Check sheet for the drawn part. Datum: minimum x, y, z corner. Units: mm. Round coordinates to 2 decimals unless told otherwise and drop trailing zeros. Write each loop counter-clockwise with the first axis right and the second up, starting at its lowest first coordinate (ties: lowest second). Pieces come first, ordered by that corner, then holes. Notation, with made-up numbers: (6, 72.25) - (53, 72.25) arc R10 ccw to (53, 76.25) - close; hole circle Ø10 at (86, 79). An arc over 180 degrees is marked (long way). Return JSON: item names as keys, results as strings. Group by question number.
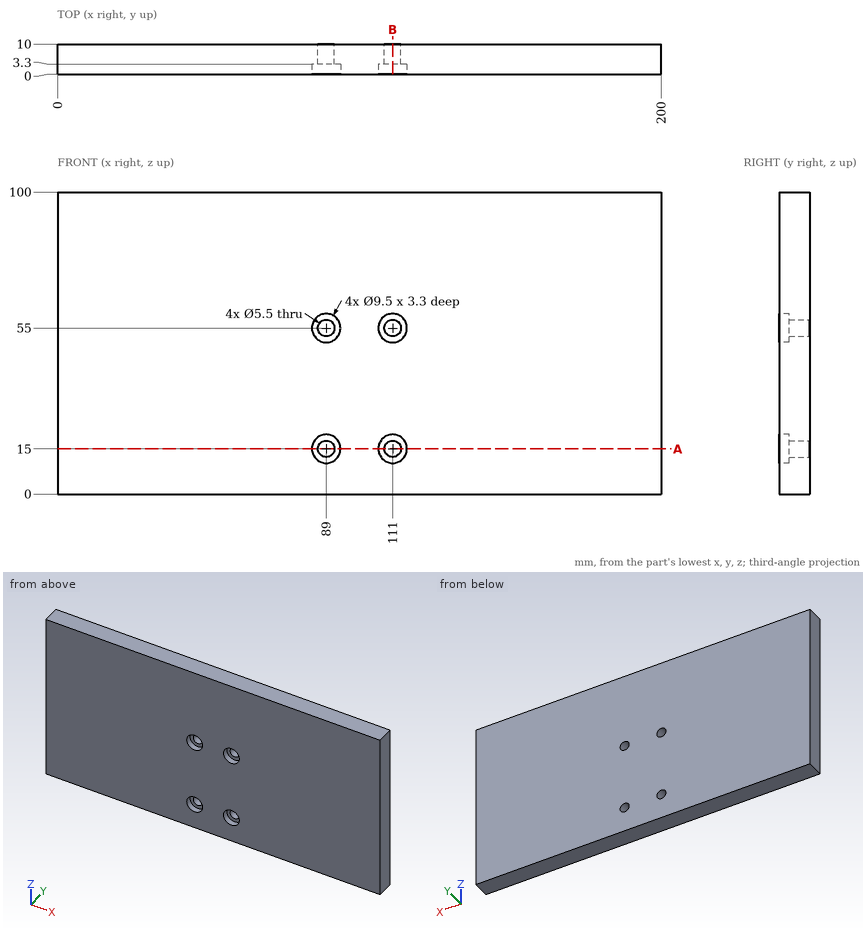
1. Section check A-A (z = 15). Enter the section's corners in (x, y).
2. Depth check by flat-ended pin: pin 1 Ø3.5 at (x, z) = (89, 55) entering from +Y; pin 2 Ø5 at (x, z) = (112, 14) entering from -Y. Enter the tip coordinate at first touch or a pass-through.
3. Material ranges on line 1 along X through (y, z) = (1, 15); line 2 along X through (y, z) = (3.5, 54); line 3 along Y through (x, z) = (113.5, 51), recorded low to high.
4. Section check B-B (x = 111). Enter the section's corners in (y, z), and give its area (3 significant figures).
Result sheet:
{
 "1": {"outline": "(0, 0) - (84.25, 0) - (84.25, 3.3) - (86.25, 3.3) - (86.25, 10) - (0, 10) - close; (91.75, 3.3) - (93.75, 3.3) - (93.75, 0) - (106.25, 0) - (106.25, 3.3) - (108.25, 3.3) - (108.25, 10) - (91.75, 10) - close; (113.75, 3.3) - (115.75, 3.3) - (115.75, 0) - (200, 0) - (200, 10) - (113.75, 10) - close"},
 "2": {"pin 1": "passes through", "pin 2": "stops at y = 3.3"},
 "3": {"line 1": "x = 0 to 84.25, 93.75 to 106.25, 115.75 to 200", "line 2": "x = 0 to 86.44, 91.56 to 108.44, 113.56 to 200", "line 3": "y = 3.3 to 10"},
 "4": {"outline": "(0, 0) - (10, 0) - (10, 12.25) - (3.3, 12.25) - (3.3, 10.25) - (0, 10.25) - close; (0, 19.75) - (3.3, 19.75) - (3.3, 17.75) - (10, 17.75) - (10, 52.25) - (3.3, 52.25) - (3.3, 50.25) - (0, 50.25) - close; (0, 59.75) - (3.3, 59.75) - (3.3, 57.75) - (10, 57.75) - (10, 100) - (0, 100) - close", "area": "864 mm²"}
}
